from build123d import *

# Parameters (mm, degrees)
SKETCH_1_R          = 3
EXTRUDE_1_DEPTH     = 1.5
SKETCH_2_R          = 2.25
EXTRUDE_2_DEPTH     = 2
SKETCH_3_R          = 1.5
CUT_EXTRUDE_1_DEPTH = 0.5
FILLET_1_R          = 0.25
FILLET_2_R          = 0.5
FILLET_3_R          = 0.5


with BuildPart() as part:
    # Эскиз1 → Бобышка-Вытянуть1 (new body)
    with BuildSketch(Plane.XY):
        Circle(SKETCH_1_R)
    extrude(amount=EXTRUDE_1_DEPTH)

    # Эскиз2 → Бобышка-Вытянуть2 (add)
    with BuildSketch(Plane.XY.offset(1.5)):
        Circle(SKETCH_2_R)
    extrude(amount=EXTRUDE_2_DEPTH)

    # Эскиз3 → Вырез-Вытянуть1 (cut)
    with BuildSketch(Plane(origin=(0, 0, 0), x_dir=(-1, 0, 0), z_dir=(0, 0, -1))):
        Circle(SKETCH_3_R)
    extrude(amount=-CUT_EXTRUDE_1_DEPTH, mode=Mode.SUBTRACT)

    # Скругление1
    fillet_1_edges = [part.edges().sort_by_distance(p)[0] for p in [
        (1.5, 0, 0.5),
    ]]
    fillet(fillet_1_edges, radius=FILLET_1_R)

    # Скругление2
    fillet_2_edges = [part.edges().sort_by_distance(p)[0] for p in [
        (-2.25, 0, 3.5),
    ]]
    fillet(fillet_2_edges, radius=FILLET_2_R)

    # Скругление3
    fillet_3_edges = [part.edges().sort_by_distance(p)[0] for p in [
        (-3, 0, 0),
    ]]
    fillet(fillet_3_edges, radius=FILLET_3_R)


solid = part.part
Geometry: final body of the model. Coordinates: model frame, mm. Coordinates: 2 decimals unless noted, no trailing zeros. Order: outer loops, then holes, each group sorted by start corner. A loop starts at its lowest first (then second) coordinate and runs counter-clockwise, first axis right, second up. Notation, with made-up numbers: M 88,-5 L 121,-5 A20 cw 121,33 Z; hole C -35,1.25 d8. An arc over 180 degrees is marked long. One line per question, with ' | ' between items. Start each with the question number.
Item 1: Ray query, probe 1 along Y at (x, z) = (0, 0.2); probe 2 along Z at (x, y) = (2.1, 1.15); probe 3 along Z at (x, y) = (1, 0.7). Return the intervals inside material, ascending. Write a range as [from, to].
Item 2: Cut plane A-A, the plane y = 0. Return the cut outline in (x, z), then the cut area to 3 significant figures.
Item 3: Draft query along X for faces 1 (the flat face through (0, -2, 0)), 2 (the cylindrical face through (-0.29, 2.23, 2.24)), 3 (the flat face through (0, 0, 0.5)). Return one class per face: released by +X, released by -X, zero draft, split by the parting line, or undercut.
Item 4: Cut plane C-C, the plane z = 1.7. Return the cut outline in (x, y).
Item 5: Pin query (flat end, axial travel): pin 1 Ø1 at (y, z) = (-2, 1) entering from -X; pin 2 Ø1.5 at (x, z) = (-1.5, 0.5) entering from -Y; pin 3 Ø1 at (x, z) = (-2, 1) entering from -Y. Return the tip coordinate at first contact, or that it passes through.
Item 6: Cut plane D-D, the plane z = 0.8. Return the cut outline in (x, y).
A:
1) probe 1: y = [-2.9, -1.5], [1.5, 2.9] | probe 2: z = [0, 1.5] | probe 3: z = [0.5, 3.5]
2) outline: M -3,0.5 A0.5 ccw -2.5,0 L -1.5,0 L -1.5,0.25 A0.25 cw -1.25,0.5 L 1.25,0.5 A0.25 cw 1.5,0.25 L 1.5,0 L 2.5,0 A0.5 ccw 3,0.5 L 3,1.5 L 2.25,1.5 L 2.25,3 A0.5 ccw 1.75,3.5 L -1.75,3.5 A0.5 ccw -2.25,3 L -2.25,1.5 L -3,1.5 Z | area: 16.3 mm2
3) face 1: zero draft | face 2: split by the parting line | face 3: undercut
4) outline: C 0,0 d4.5
5) pin 1: stops at x = -2.6 | pin 2: stops at y = -2.9 | pin 3: stops at y = -2.6
6) outline: C 0,0 d6
